from build123d import *

# Parameters (mm, degrees)
SKETCH_1_R      = 28
SKETCH_1_R_2    = 4.25
SKETCH_1_R_3    = 1.5
EXTRUDE_1_DEPTH = 4


with BuildPart() as part:
    # 草图1 → 凸台-拉伸1 (new body)
    with BuildSketch(Plane.XY):
        Circle(SKETCH_1_R)
        Circle(SKETCH_1_R_2, mode=Mode.SUBTRACT)
        with Locations((12.5, 21.650635095)):
            Circle(SKETCH_1_R_3, mode=Mode.SUBTRACT)
        with Locations((25, 0)):
            Circle(SKETCH_1_R_3, mode=Mode.SUBTRACT)
        with Locations((12.5, -21.650635095)):
            Circle(SKETCH_1_R_3, mode=Mode.SUBTRACT)
        with Locations((-12.5, -21.650635095)):
            Circle(SKETCH_1_R_3, mode=Mode.SUBTRACT)
        with Locations((-25, 0)):
            Circle(SKETCH_1_R_3, mode=Mode.SUBTRACT)
        with Locations((-12.5, 21.650635095)):
            Circle(SKETCH_1_R_3, mode=Mode.SUBTRACT)
        with BuildLine():
            ThreePointArc((9.006664199, -5.2), (15.290381057, -3.516283143), (16.974097914, -9.8))
            ThreePointArc((16.974097914, -9.8), (9.8, -16.974097914), (0, -19.6))
            ThreePointArc((0, -19.6), (-4.6, -15), (0, -10.4))
            ThreePointArc((0, -10.4), (5.2, -9.006664199), (9.006664199, -5.2))
        make_face(mode=Mode.SUBTRACT)
        with BuildLine():
            ThreePointArc((-9.006664199, 5.2), (-10.4, 0), (-9.006664199, -5.2))
            ThreePointArc((-9.006664199, -5.2), (-10.690381057, -11.483716857), (-16.974097914, -9.8))
            ThreePointArc((-16.974097914, -9.8), (-19.6, 0), (-16.974097914, 9.8))
            ThreePointArc((-16.974097914, 9.8), (-10.690381057, 11.483716857), (-9.006664199, 5.2))
        make_face(mode=Mode.SUBTRACT)
        with BuildLine():
            ThreePointArc((9.006664199, 5.2), (5.2, 9.006664199), (0, 10.4))
            ThreePointArc((0, 10.4), (-4.6, 15), (0, 19.6))
            ThreePointArc((0, 19.6), (9.8, 16.974097914), (16.974097914, 9.8))
            ThreePointArc((16.974097914, 9.8), (15.290381057, 3.516283143), (9.006664199, 5.2))
        make_face(mode=Mode.SUBTRACT)
    extrude(amount=EXTRUDE_1_DEPTH)


solid = part.part
Geometry: final body of the model. Coordinates: model frame, mm. A direction names the side the tool comes from. Coordinates: 2 decimals unless noted, no trailing zeros. Order: outer loops, then holes, each group sorted by start corner. A loop starts at its lowest first (then second) coordinate and runs counter-clockwise, first axis right, second up.
1) Section C-C (x = 13). Return loops of the section in (y, z), then the cut area to 3 significant figures.
Result sheet:
outline: (-24.8, 0) - (-23.06, 0) - (-23.06, 4) - (-24.8, 4) - close; (-20.24, 0) - (-14.67, 0) - (-14.67, 4) - (-20.24, 4) - close; (-2.9, 0) - (2.9, 0) - (2.9, 4) - (-2.9, 4) - close; (14.67, 0) - (20.24, 0) - (20.24, 4) - (14.67, 4) - close; (23.06, 0) - (24.8, 0) - (24.8, 4) - (23.06, 4) - close
area: 81.6 mm2
2) Set-up query: faces 4 (the flat face through (6, 0, 0)), 5 (the cylindrical face through (-10.4, 0.1, 2)). Return all of +Z, -Z, +X, -X, +Y, -Y with unobstructed straight access to the full face (end or side cutting, diameter ignored); none if empty.
Result sheet:
face 4: -Z, +X, -X, +Y, -Y
face 5: +Z, -Z
3) Ray query, probe 1 along Y at (x, z) = (-12.5, 2.55); probe 2 along Y at (x, z) = (5, 1.85); probe 3 along X at (y, z) = (-2.5, 0.65). Return the intervals inside material, ascending.
Result sheet:
probe 1: y = -25.05 to -23.15, -20.15 to -12.07, 12.07 to 20.15, 23.15 to 25.05
probe 2: y = -27.55 to -18.95, -9.12 to 9.12, 18.95 to 27.55
probe 3: x = -27.89 to -19.44, -10.1 to -3.44, 3.44 to 27.89
4) Draft query along X for faces 1 (the cylindrical face through (25.865, -10.724, 1.972)), 2 (the flat face through (6, 0, 4)), 3 (the cylindrical face through (15.202, -3.467, 1.972)). Return one class per face: released by +X, released by -X, zero draft, split by the parting line, or undercut.
Result sheet:
face 1: split by the parting line
face 2: zero draft
face 3: undercut
5) Section B-B (x = -2.5). Return loops of the section in (y, z).
Result sheet:
outline: (-27.89, 0) - (-18.86, 0) - (-18.86, 4) - (-27.89, 4) - close; (-11.14, 0) - (-3.44, 0) - (-3.44, 4) - (-11.14, 4) - close; (3.44, 0) - (11.14, 0) - (11.14, 4) - (3.44, 4) - close; (18.86, 0) - (27.89, 0) - (27.89, 4) - (18.86, 4) - close
6) Section A-A (y = 0). Return loops of the section in (x, z).
Result sheet:
outline: (-28, 0) - (-26.5, 0) - (-26.5, 4) - (-28, 4) - close; (-23.5, 0) - (-19.6, 0) - (-19.6, 4) - (-23.5, 4) - close; (-10.4, 0) - (-4.25, 0) - (-4.25, 4) - (-10.4, 4) - close; (4.25, 0) - (23.5, 0) - (23.5, 4) - (4.25, 4) - close; (26.5, 0) - (28, 0) - (28, 4) - (26.5, 4) - close
7) Section D-D (y = -15). Return loops of the section in (x, z), then the cut area to 3 significant figures.
Result sheet:
outline: (-23.64, 0) - (-4.6, 0) - (-4.6, 4) - (-23.64, 4) - close; (12.62, 0) - (23.64, 0) - (23.64, 4) - (12.62, 4) - close
area: 120 mm2
